Check sheet for the modelled part. Datum: model origin and axes. Units: mm. A direction names the side the tool comes from. Coordinates: 2 decimals unless noted, no trailing zeros. Loops run counter-clockwise (first coordinate to the right, second up) from the corner with the lowest first, then second, coordinate; pieces in that order, holes last. Notation, with made-up numbers: (-19, -39.5) - (10, -39.5) arc R23 cw to (10, -17.5) - close; hole circle Ø3 at (37, -17). An arc over 180 degrees is marked (long way). Use a Markdown table: item, result. Add a question column.
1) Sectioned sample at D-D, the plane x = -22. Enter the section's corners in (y, z).
2) Thickness scan on line 1 (Z direction, x = -25, y = 1); line 2 (Y direction, x = -3.5, z = -0.95); line 3 (X direction, y = 27, z = -1). Record the ranges inside material, lowest first.
3) Tool access check on faces 1 (the cylindrical face through (-0.91, 34.95, -0.7)), 2 (the flat face through (0, -37.5, 0)), 3 (the cylindrical face through (-0.91, -35.02, -0.7)). Record the directions out of +Z, -Z, +X, -X, +Y, -Y that give a thin tool (end or side, any length) a straight path to the whole face; none if there is none.
4) Go/stop test with flat-tipped pins: P1, Ø6, axis at x = -25.5, y = 27.5, coming from the -Z side; P2, Ø2, axis at y = 21, z = 0, coming from the -X side; P3, Ø5, axis at x = 19, y = 1.5, coming from the +Z side; P4, Ø6, axis at x = -7.5, y = 0, coming from the -Z side. Record where each tip stops, or that it passes through.
5) Sectioned sample at B-B, the plane x = 20.5. Enter the section's corners in (y, z).
6) Sectioned sample at C-C, the plane y = 31.5. Enter the section's corners in (x, z), then the cut area to 3 significant figures.
7) Sectioned sample at A-A, the plane y = 0. Enter the section's corners in (x, z).
from build123d import *

# Parameters (mm, degrees)
F1_DEPTH = 32.5
F2_W     = 70
F2_H     = 70
F2_R     = 32.5
F3_DEPTH = 5
F5_R     = 1.15
F6_DEPTH = 37.5


with BuildPart() as f1:
    # F0 (on Front) → F1 (new body, symmetric)
    with BuildSketch(Plane.XZ):
        Polygon((0, 2.5), (-32.5, 0.75), (-32.5, -0.75), (0, -2.5), (32.5, -0.75), (32.5, 0.75), align=None)
    extrude(amount=F1_DEPTH, both=True)


with BuildPart() as f3:
    # F2 (on Top) → F3 (new body, symmetric)
    with BuildSketch(Plane.XY):
        Rectangle(F2_W, F2_H)
        Circle(F2_R, mode=Mode.SUBTRACT)
    extrude(amount=F3_DEPTH, both=True)


with BuildPart() as f1_1:
    add(f1.part)

    # F4: cut F3
    add(f3.part, mode=Mode.SUBTRACT)

    # F5 (on Front) → F6 (join, symmetric)
    with BuildSketch(Plane.XZ):
        Circle(F5_R)
    extrude(amount=F6_DEPTH, both=True)


solid = f1_1.part
Solved:
| question | item | result |
|---|---|---|
| 1 | outline | (-23.92, -1.32) - (23.92, -1.32) - (23.92, 1.32) - (-23.92, 1.32) - close |
| 2 | line 1 | z = -1.15 to 1.15 |
| 2 | line 2 | y = -32.31 to 32.31 |
| 2 | line 3 | x = -18.09 to 18.09 |
| 3 | face 1 | +Y |
| 3 | face 2 | +Z, -Z, +X, -X, -Y |
| 3 | face 3 | -Y |
| 4 | P1 | passes through |
| 4 | P2 | stops at x = -25.62 |
| 4 | P3 | stops at z = 1.61 |
| 4 | P4 | stops at z = -2.26 |
| 5 | outline | (-25.22, -1.4) - (25.22, -1.4) - (25.22, 1.4) - (-25.22, 1.4) - close |
| 6 | outline | (-8, -2.07) - (0, -2.5) - (8, -2.07) - (8, 2.07) - (0, 2.5) - (-8, 2.07) - close |
| 6 | area | 73.1 mm2 |
| 7 | outline | (-32.5, -0.75) - (0, -2.5) - (32.5, -0.75) - (32.5, 0.75) - (0, 2.5) - (-32.5, 0.75) - close |
